Part model, mm, in its own coordinate system. A direction names the side the tool comes from. Coordinates: 2 decimals unless noted, no trailing zeros. Loops run counter-clockwise (first coordinate to the right, second up) from the corner with the lowest first, then second, coordinate; pieces in that order, holes last. Notation, with made-up numbers: M -32,4 L -25,4 A24 ccw -25,28 Z; hole C 43,43 d6. An arc over 180 degrees is marked long. Answer as a JSON object with one key per item and string values. Group by question number.
1. Drop flat-ended pins along their axis: pin 1 Ø0.7 at (x, z) = (-0.5, 19.5) entering from +Y; pin 2 Ø0.8 at (y, z) = (-9, 1.5) entering from -X; pin 3 Ø2.5 at (y, z) = (-0.5, 15.5) entering from +X. Give the stop position or say it passes through.
2. 3-axis set-ups, long thin cutter, end or side, ignore diameter. For faces 4 (the face through (-2.256, 3.835, 0.63)), 5 (the face through (-3.6, 0, 1)), 6 (the face through (0, -3.6, 1)): which of +Z, -Z, +X, -X, +Y, -Y reach the whole face in a straight line?
3. Drill centre lines: L1, parallel to Y at x = 0, z = 13; L2, parallel to Y at x = -3.25, z = 16.5; L3, parallel to Y at x = 2.75, z = -25. Where is each one in solid material? Low to high.
4. Mould opens along X. For faces 1 (the face through (-4, -8.2, 1)), 2 (the face through (0.1, 2.4, -45)), 3 (the face through (3.6, 0, 1)) say: released by +X, released by -X, zero draft, split by the parting line, or undercut.
5. Saw through at A-A on y = 0. Write the cut outline in (x, z), then the cut area to 3 significant figures.
from build123d import *

# Parameters (mm, degrees)
SKETCH3_R                = 2.15
BOSS_EXTRUDE1_DEPTH      = 45
BOSS_EXTRUDE1_DEPTH_BACK = 45


with BuildPart() as part:
    # Sketch3 → Boss-Extrude1 (new body, two sides)
    with BuildSketch(Plane.XY) as boss_extrude1_sk:
        with BuildLine():
            Line((3.2874, 10), (8, 10))
            ThreePointArc((8, 10), (9.414213562, 9.414213562), (10, 8))
            Line((10, 8), (10, 3.2874))
            ThreePointArc((10, 3.2874), (9.76937588, 2.73062412), (9.2126, 2.5))
            Line((9.2126, 2.5), (8.5048, 2.5))
            ThreePointArc((8.5048, 2.5), (8.289273853, 2.589273853), (8.2, 2.8048))
            Line((8.2, 2.8048), (8.2, 4.9118))
            ThreePointArc((8.2, 4.9118), (7.682565253, 5.686195824), (6.769103096, 5.504496904))
            Line((6.769103096, 5.504496904), (4.478679656, 3.214073464))
            ThreePointArc((4.478679656, 3.214073464), (3.828361402, 2.240803418), (3.6, 1.092753121))
            Line((3.6, 1.092753121), (3.6, -1.092753121))
            ThreePointArc((3.6, -1.092753121), (3.828361402, -2.240803418), (4.478679656, -3.214073464))
            Line((4.478679656, -3.214073464), (6.769103096, -5.504496904))
            ThreePointArc((6.769103096, -5.504496904), (7.682565253, -5.686195824), (8.2, -4.9118))
            Line((8.2, -4.9118), (8.2, -2.8048))
            ThreePointArc((8.2, -2.8048), (8.289273853, -2.589273853), (8.5048, -2.5))
            Line((8.5048, -2.5), (9.2126, -2.5))
            ThreePointArc((9.2126, -2.5), (9.76937588, -2.73062412), (10, -3.2874))
            Line((10, -3.2874), (10, -8))
            ThreePointArc((10, -8), (9.414213562, -9.414213562), (8, -10))
            Line((8, -10), (3.2874, -10))
            ThreePointArc((3.2874, -10), (2.73062412, -9.76937588), (2.5, -9.2126))
            Line((2.5, -9.2126), (2.5, -8.5048))
            ThreePointArc((2.5, -8.5048), (2.589273853, -8.289273853), (2.8048, -8.2))
            Line((2.8048, -8.2), (4.9118, -8.2))
            ThreePointArc((4.9118, -8.2), (5.686195824, -7.682565253), (5.504496904, -6.769103096))
            Line((5.504496904, -6.769103096), (3.214073464, -4.478679656))
            ThreePointArc((3.214073464, -4.478679656), (2.240803418, -3.828361402), (1.092753121, -3.6))
            Line((1.092753121, -3.6), (-1.092753121, -3.6))
            ThreePointArc((-1.092753121, -3.6), (-2.240803418, -3.828361402), (-3.214073464, -4.478679656))
            Line((-3.214073464, -4.478679656), (-5.504496904, -6.769103096))
            ThreePointArc((-5.504496904, -6.769103096), (-5.686195824, -7.682565253), (-4.9118, -8.2))
            Line((-4.9118, -8.2), (-2.8048, -8.2))
            ThreePointArc((-2.8048, -8.2), (-2.589273853, -8.289273853), (-2.5, -8.5048))
            Line((-2.5, -8.5048), (-2.5, -9.2126))
            ThreePointArc((-2.5, -9.2126), (-2.73062412, -9.76937588), (-3.2874, -10))
            Line((-3.2874, -10), (-8, -10))
            ThreePointArc((-8, -10), (-9.414213562, -9.414213562), (-10, -8))
            Line((-10, -8), (-10, -3.2874))
            ThreePointArc((-10, -3.2874), (-9.76937588, -2.73062412), (-9.2126, -2.5))
            Line((-9.2126, -2.5), (-8.5048, -2.5))
            ThreePointArc((-8.5048, -2.5), (-8.289273853, -2.589273853), (-8.2, -2.8048))
            Line((-8.2, -2.8048), (-8.2, -4.9118))
            ThreePointArc((-8.2, -4.9118), (-7.682565253, -5.686195824), (-6.769103096, -5.504496904))
            Line((-6.769103096, -5.504496904), (-4.478679656, -3.214073464))
            ThreePointArc((-4.478679656, -3.214073464), (-3.828361402, -2.240803418), (-3.6, -1.092753121))
            Line((-3.6, -1.092753121), (-3.6, 1.092753121))
            ThreePointArc((-3.6, 1.092753121), (-3.828361402, 2.240803418), (-4.478679656, 3.214073464))
            Line((-4.478679656, 3.214073464), (-6.769103096, 5.504496904))
            ThreePointArc((-6.769103096, 5.504496904), (-7.682565253, 5.686195824), (-8.2, 4.9118))
            Line((-8.2, 4.9118), (-8.2, 2.8048))
            ThreePointArc((-8.2, 2.8048), (-8.289273853, 2.589273853), (-8.5048, 2.5))
            Line((-8.5048, 2.5), (-9.2126, 2.5))
            ThreePointArc((-9.2126, 2.5), (-9.76937588, 2.73062412), (-10, 3.2874))
            Line((-10, 3.2874), (-10, 8))
            ThreePointArc((-10, 8), (-9.414213562, 9.414213562), (-8, 10))
            Line((-8, 10), (-3.2874, 10))
            ThreePointArc((-3.2874, 10), (-2.73062412, 9.76937588), (-2.5, 9.2126))
            Line((-2.5, 9.2126), (-2.5, 8.5048))
            ThreePointArc((-2.5, 8.5048), (-2.589273853, 8.289273853), (-2.8048, 8.2))
            Line((-2.8048, 8.2), (-4.9118, 8.2))
            ThreePointArc((-4.9118, 8.2), (-5.686195824, 7.682565253), (-5.504496904, 6.769103096))
            Line((-5.504496904, 6.769103096), (-3.214073464, 4.478679656))
            ThreePointArc((-3.214073464, 4.478679656), (-2.240803418, 3.828361402), (-1.092753121, 3.6))
            Line((-1.092753121, 3.6), (1.092753121, 3.6))
            ThreePointArc((1.092753121, 3.6), (2.240803418, 3.828361402), (3.214073464, 4.478679656))
            Line((3.214073464, 4.478679656), (5.504496904, 6.769103096))
            ThreePointArc((5.504496904, 6.769103096), (5.686195824, 7.682565253), (4.9118, 8.2))
            Line((4.9118, 8.2), (2.8048, 8.2))
            ThreePointArc((2.8048, 8.2), (2.589273853, 8.289273853), (2.5, 8.5048))
            Line((2.5, 8.5048), (2.5, 9.2126))
            ThreePointArc((2.5, 9.2126), (2.73062412, 9.76937588), (3.2874, 10))
        make_face()
        Circle(SKETCH3_R, mode=Mode.SUBTRACT)
    extrude(amount=BOSS_EXTRUDE1_DEPTH)
    extrude(boss_extrude1_sk.sketch, amount=-BOSS_EXTRUDE1_DEPTH_BACK)


solid = part.part
Outcome:
{
 "1": {"pin 1": "stops at y = 3.6", "pin 2": "stops at x = -9.91", "pin 3": "stops at x = 3.67"},
 "2": {"face 4": "+Z, -Z", "face 5": "+Z, -Z, -X", "face 6": "+Z, -Z, -Y"},
 "3": {"L1": "y = -3.6 to -2.15, 2.15 to 3.6", "L2": "y = -10 to -8.2, -4.51 to 4.51, 8.2 to 10", "L3": "y = -9.79 to -8.2, -4.1 to 4.1, 8.2 to 9.79"},
 "4": {"face 1": "undercut", "face 2": "zero draft", "face 3": "released by +X"},
 "5": {"outline": "M -3.6,-45 L -2.15,-45 L -2.15,45 L -3.6,45 Z; M 2.15,-45 L 3.6,-45 L 3.6,45 L 2.15,45 Z", "area": "261 mm²"}
}
